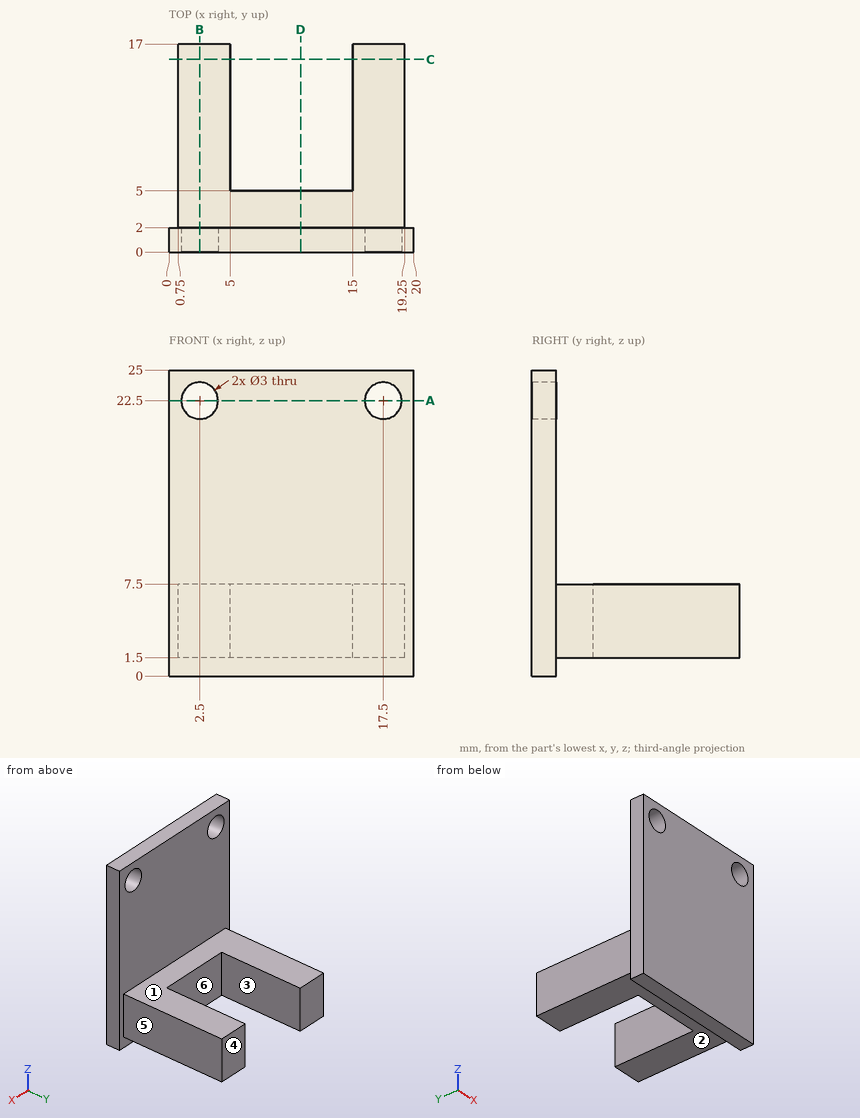
Drawing for the job (mm, zero at the part's lowest x, y, z). A direction names the side the tool comes from. Round coordinates to 2 decimals unless told otherwise and drop trailing zeros. Write each loop counter-clockwise with the first axis right and the second up, starting at its lowest first coordinate (ties: lowest second). Pieces come first, ordered by that corner, then holes. Notation, with made-up numbers: M 62.25,25.25 L 118.25,25.25 A22 ccw 118.25,35.25 Z; hole C 13.5,-19 d1. An arc over 180 degrees is marked long. Answer as a JSON object with one key per item and string values. Group by question number.
(1) Flat gauge pins, fed straight in: pin 1 (1.8 mm diameter, centred on x = 7.5, z = 5, fed in from +Y); pin 2 (1.5 mm diameter, centred on x = 6.5, y = 4, fed in from +Z); pin 3 (4 mm diameter, centred on x = 2.5, z = 22.5, fed in from +Y). Where does each tip first touch, or does it go through?
(2) Which spindle directions (+Z, -Z, +X, -X, +Y, -Y) get a long thin tool onto all of the face, cutting with end or side? Do the marked faces 1, 2 and 3. Say none if no direction does.
(3) Cut at C-C (y = 15.75). Give the cut face in (x, z), and give its area (3 significant figures).
(4) Mould opens along X. For the marked faces 4, 5 and 6 say: pulls with the +X half, pulls with the -X half, needs draft (parallel to the pull), parting line crosses it, or undercut.
(5) Cut at A-A (z = 22.5). Give the cut face in (x, y).
(6) Cut at B-B (x = 2.5). Give the cut face in (y, z).
(7) Cut at D-D (x = 10.75). Give the cut face in (y, z).
(8) Drill centre lines: L1, parallel to X at y = 0.8, z = 22.5; L2, parallel to Z at x = 17.5, y = 1.05; L3, parallel to Y at x = 9, z = 2.5. Where is each one in solid material? Low to high.
Responses:
{
 "1": {"pin 1": "stops at y = 5", "pin 2": "stops at z = 7.5", "pin 3": "stops at y = 2"},
 "2": {"face 1": "+Z, +X, -X, +Y", "face 2": "-Z, +X, -X, +Y", "face 3": "+Z, -Z, +Y"},
 "3": {"outline": "M 0.75,1.5 L 5,1.5 L 5,7.5 L 0.75,7.5 Z; M 15,1.5 L 19.25,1.5 L 19.25,7.5 L 15,7.5 Z", "area": "51.0 mm2"},
 "4": {"face 4": "needs draft", "face 5": "pulls with the +X half", "face 6": "undercut"},
 "5": {"outline": "M 0,0 L 1,0 L 1,2 L 0,2 Z; M 4,0 L 16,0 L 16,2 L 4,2 Z; M 19,0 L 20,0 L 20,2 L 19,2 Z"},
 "6": {"outline": "M 0,0 L 2,0 L 2,1.5 L 17,1.5 L 17,7.5 L 2,7.5 L 2,21 L 0,21 Z; M 0,24 L 2,24 L 2,25 L 0,25 Z"},
 "7": {"outline": "M 0,0 L 2,0 L 2,1.5 L 5,1.5 L 5,7.5 L 2,7.5 L 2,25 L 0,25 Z"},
 "8": {"L1": "x = 0 to 1, 4 to 16, 19 to 20", "L2": "z = 0 to 21, 24 to 25", "L3": "y = 0 to 5"}
}
